```python
from build123d import *

# Parameters (mm, degrees)
SALIENTE_EXTRUIR1_DEPTH           = 325
TALADRO3_DEPTH                    = 6.35
TALADRO_DE_MARGEN_PARA_M561_D     = 62
TALADRO_DE_MARGEN_PARA_M561_DEPTH = 287.94
TALADRO_DE_MARGEN_PARA_M561_TIP   = 18.62667919


# Read off the part's stored shape, not the designer's step: Taladro3
with BuildPart() as part:
    # Croquis1 → Saliente-Extruir1 (new, symmetric)
    with BuildSketch(Plane.XY):
        Polygon((0, 0), (0, 65), (6.35, 65), (6.35, 6.35), (65, 6.35), (65, 0), align=None)
    extrude(amount=SALIENTE_EXTRUIR1_DEPTH, both=True)

    # Taladro3 outline → Taladro3 (cut)
    with BuildSketch(Plane.YZ):
        with BuildLine():
            Line((65, 204.912035309), (65, 256.022124888))
            ThreePointArc((65, 256.022124888), (27.341767585, 230.467080098), (65, 204.912035309))
        make_face()
    extrude(amount=TALADRO3_DEPTH, mode=Mode.SUBTRACT)

    # Taladro de margen para M561
    with Locations(Plane(origin=(6.35, 55.113874636, 289.004791986), x_dir=(0, 1, 0), z_dir=(1, 0, 0))):
        with Locations((1.236125364, -461.004791986)):
            Hole(TALADRO_DE_MARGEN_PARA_M561_D / 2, depth=TALADRO_DE_MARGEN_PARA_M561_DEPTH)
            with Locations((0, 0, -(TALADRO_DE_MARGEN_PARA_M561_DEPTH + TALADRO_DE_MARGEN_PARA_M561_TIP / 2))):  # 118° drill point
                Cone(0, TALADRO_DE_MARGEN_PARA_M561_D / 2, TALADRO_DE_MARGEN_PARA_M561_TIP, mode=Mode.SUBTRACT)


solid = part.part
```
Verification items for the finished model (mm, model axes). A direction names the side the tool comes from. Give positions to 0.01 mm unless a question says otherwise; leave off trailing zeros. Write each loop counter-clockwise with the first axis right and the second up, starting at its lowest first coordinate (ties: lowest second). Pieces come first, ordered by that corner, then holes. Notation, with made-up numbers: (48.25, -13) - (87.25, -13) arc R17 ccw to (87.25, 6) - close; hole circle Ø5 at (88.5, -1). An arc over 180 degrees is marked (long way). Put each result on its own line as item: value.
Q1. Section check B-B on z = -172. Record the cut outline in (x, y).
Result:
outline: (0, 0) - (65, 0) - (65, 6.35) - (6.35, 6.35) - (6.35, 25.35) - (0, 25.35) - close
Q2. Section check A-A on y = 56.35. Record the cut outline in (x, z).
Result:
outline: (0, -325) - (6.35, -325) - (6.35, -203) - (0, -203) - close; (0, -141) - (6.35, -141) - (6.35, 203.01) - (0, 203.01) - close; (0, 257.93) - (6.35, 257.93) - (6.35, 325) - (0, 325) - close
Q3. Section check C-C on x = 18. Record the cut outline in (y, z).
Result:
outline: (0, -325) - (6.35, -325) - (6.35, 325) - (0, 325) - close
Q4. Section check D-D on z = 249.5. Record the cut outline in (x, y).
Result:
outline: (0, 0) - (65, 0) - (65, 6.35) - (6.35, 6.35) - (6.35, 34.99) - (0, 34.99) - close
Q5. Depth check by flat-ended pin: P1, Ø6, axis at x = 18.5, z = 169.5, coming from the +Y side; P2, Ø10, axis at y = 15, z = -250.5, coming from the +X side. Enter the tip coordinate at first touch or a pass-through.
Result:
P1: y = 6.35
P2: x = 6.35
Q6. Mould release check, pull along Z, two halves, no side actions. Record for faces 3 (the face through (3.13, 25.36, -172.8)), 4 (the face through (18, 6, -325)), 5 (the face through (18, 6, 325)): released by +Z, released by -Z, zero draft, split by the parting line, or undercut.
Result:
face 3: undercut
face 4: released by -Z
face 5: released by +Z
Q7. Scan lines: probe 1 along Z at (x, y) = (4.75, 56.35); probe 2 along X at (y, z) = (20, -116.5); probe 3 along Y at (x, z) = (5, -172). Record each from-to range of solid material in increasing order. Write a range as from..to.
Result:
probe 1: -325..-203, -141..203.01, 257.93..325
probe 2: 0..6.35
probe 3: 0..25.35
Q8. Set-up check for faces 1 (the face through (33, 0, 5)), 2 (the face through (35, 6.35, 5)): record each of +Z, -Z, +X, -X, +Y, -Y from which the full face is reachable in a straight line by a thin tool's end or side.
Result:
face 1: +Z, -Z, +X, -X, -Y
face 2: +Z, -Z, +X, +Y
